Geometry: see drawing. Coordinates: mm, zero at the bounding-box minimum. A direction names the side the tool comes from. Give positions to 0.01 mm unless a question says otherwise; leave off trailing zeros. Order: outer loops, then holes, each group sorted by start corner. A loop starts at its lowest first (then second) coordinate and runs counter-clockwise, first axis right, second up. Notation, with made-up numbers: M -15.5,39.25 L 37.5,39.25 A18 ccw 37.5,63.25 Z; hole C -21,-12 d9. An arc over 180 degrees is marked long. Return JSON: item names as keys, results as strings.
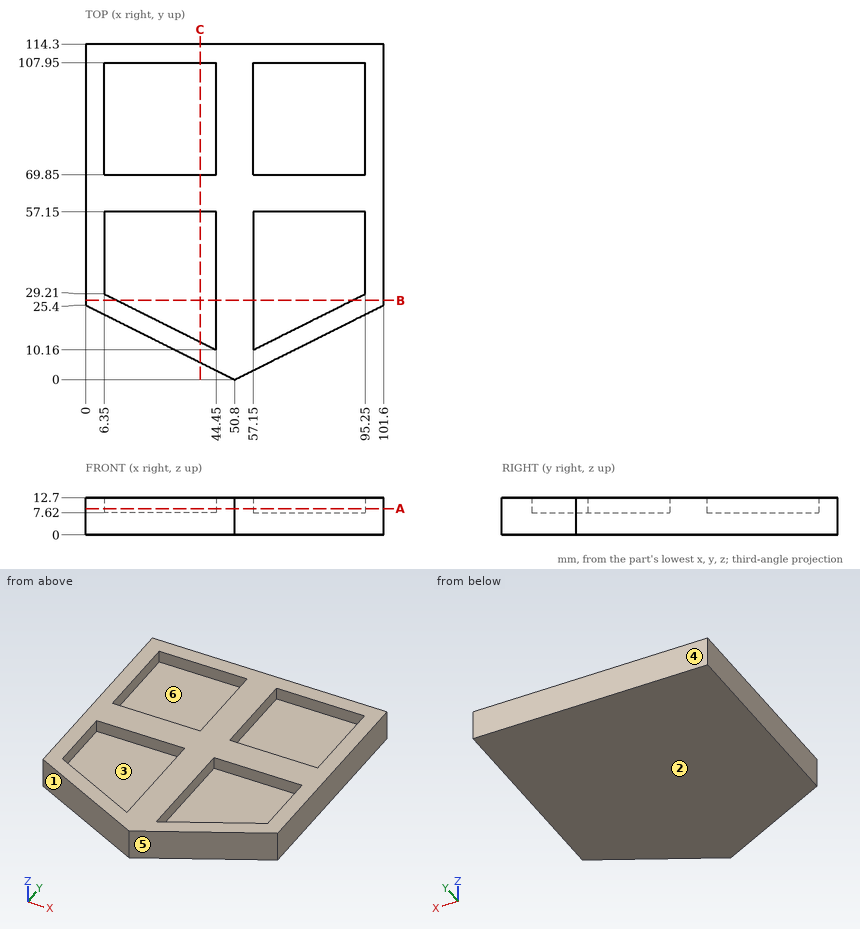
1. Ray query, probe 1 along X at (y, z) = (95, 11.25); probe 2 along Y at (x, z) = (76, 12) (3 decimals). Return the intervals inside material, ascending.
Evaluation:
{"probe 1": "x = 0 to 6.35, 44.45 to 57.15, 95.25 to 101.6", "probe 2": "y = 12.6 to 19.585, 57.15 to 69.85, 107.95 to 114.3"}
2. Section query B-B (y = 27). Return loops of the section in (x, z).
Evaluation:
{"outline": "M 0,0 L 101.6,0 L 101.6,12.7 L 90.83,12.7 L 90.83,7.62 L 57.15,7.62 L 57.15,12.7 L 44.45,12.7 L 44.45,7.62 L 10.77,7.62 L 10.77,12.7 L 0,12.7 Z"}
3. First-contact query: pin 1 (5.5 mm diameter, centred on x = 81, z = 10.5, fed in from -Y) (3 decimals); pin 2 (5.5 mm diameter, centred on x = 19.5, z = 9, fed in from -Y) (3 decimals); pin 3 (11.5 mm diameter, centred on x = 26.5, y = 44, fed in from +Z). Flat tips, straight axial feed; report the tip coordinate or a pass-through.
Evaluation:
{"pin 1": "stops at y = 13.725", "pin 2": "stops at y = 14.275", "pin 3": "stops at z = 7.62"}
4. Section query A-A (z = 9). Return loops of the section in (x, y), then the cut area to 3 significant figures.
Evaluation:
{"outline": "M 0,25.4 L 50.8,0 L 101.6,25.4 L 101.6,114.3 L 0,114.3 Z; hole M 6.35,29.21 L 44.45,10.16 L 44.45,57.15 L 6.35,57.15 Z; hole M 6.35,69.85 L 44.45,69.85 L 44.45,107.95 L 6.35,107.95 Z; hole M 57.15,10.16 L 95.25,29.21 L 95.25,57.15 L 57.15,57.15 Z; hole M 57.15,69.85 L 95.25,69.85 L 95.25,107.95 L 57.15,107.95 Z", "area": "4,560 mm^2"}
5. Set-up query: the marked faces 5 and 6. Return all of +Z, -Z, +X, -X, +Y, -Y with unobstructed straight access to the full face (end or side cutting, diameter ignored); none if empty.
Evaluation:
{"face 5": "+Z, -Z, +X, -Y", "face 6": "+Z"}
6. Draft query along Y for the marked faces 1, 2, 3 and 4. Return one class per face: pulls with the +Y half, pulls with the -Y half, needs draft (parallel to the pull), parting line crosses it, or undercut.
Evaluation:
{"face 1": "pulls with the -Y half", "face 2": "needs draft", "face 3": "undercut", "face 4": "pulls with the +Y half"}
7. Section query C-C (x = 39). Return loops of the section in (y, z) (3 decimals).
Evaluation:
{"outline": "M 5.9,0 L 114.3,0 L 114.3,12.7 L 107.95,12.7 L 107.95,7.62 L 69.85,7.62 L 69.85,12.7 L 57.15,12.7 L 57.15,7.62 L 12.885,7.62 L 12.885,12.7 L 5.9,12.7 Z"}
